```python
from build123d import *

# Parameters (mm, degrees)
SKETCH1_W           = 61
SKETCH1_H           = 101
BOSS_EXTRUDE1_DEPTH = 2
SKETCH2_W           = 65
SKETCH2_H           = 105
BOSS_EXTRUDE2_DEPTH = 2.5
SKETCH4_R           = 3
SKETCH4_R_2         = 1.5
BOSS_EXTRUDE3_DEPTH = 5
SKETCH5_W           = 25
SKETCH5_H           = 32
CUT_EXTRUDE1_DEPTH  = 2
SKETCH6_W           = 2
SKETCH6_H           = 4
CUT_EXTRUDE2_DEPTH  = 3
CUT_EXTRUDE3_DEPTH  = 2.5


with BuildPart() as part:
    # Sketch1 → Boss-Extrude1 (new body)
    with BuildSketch(Plane(origin=(0, 0, 0), x_dir=(1, 0, 0), z_dir=(0, 1, 0))):
        Rectangle(SKETCH1_W, SKETCH1_H)
    extrude(amount=BOSS_EXTRUDE1_DEPTH)

    # Sketch2 → Boss-Extrude2 (add)
    with BuildSketch(Plane(origin=(0, 2, 0), x_dir=(1, 0, 0), z_dir=(0, 1, 0))):
        Rectangle(SKETCH2_W, SKETCH2_H)
    extrude(amount=BOSS_EXTRUDE2_DEPTH)

    # Sketch4 → Boss-Extrude3 (add)
    with BuildSketch(Plane(origin=(0, 4.5, 0), x_dir=(1, 0, 0), z_dir=(0, 1, 0))):
        with Locations((-9, -7.5)):
            Circle(SKETCH4_R)
        with Locations((-9, -7.5)):
            Circle(SKETCH4_R_2, mode=Mode.SUBTRACT)
        with Locations((9, -7.5)):
            Circle(SKETCH4_R)
        with Locations((9, -7.5)):
            Circle(SKETCH4_R_2, mode=Mode.SUBTRACT)
        with Locations((9, 38.5)):
            Circle(SKETCH4_R)
        with Locations((9, 38.5)):
            Circle(SKETCH4_R_2, mode=Mode.SUBTRACT)
        with Locations((-9, 38.5)):
            Circle(SKETCH4_R)
        with Locations((-9, 38.5)):
            Circle(SKETCH4_R_2, mode=Mode.SUBTRACT)
    extrude(amount=BOSS_EXTRUDE3_DEPTH)

    # Sketch5 → Cut-Extrude1 (cut)
    with BuildSketch(Plane(origin=(0, 4.5, 0), x_dir=(1, 0, 0), z_dir=(0, 1, 0))):
        with Locations((0, -48.5)):
            Rectangle(SKETCH5_W, SKETCH5_H)
    extrude(amount=-CUT_EXTRUDE1_DEPTH, mode=Mode.SUBTRACT)

    # Sketch6 → Cut-Extrude2 (cut)
    with BuildSketch(Plane(origin=(0, 9.5, 0), x_dir=(1, 0, 0), z_dir=(0, 1, 0))):
        with Locations((9, -6)):
            Rectangle(SKETCH6_W, SKETCH6_H)
        with Locations((-9, -6)):
            Rectangle(SKETCH6_W, SKETCH6_H)
        with Locations((9, 37)):
            Rectangle(SKETCH6_W, SKETCH6_H)
        with Locations((-9, 37)):
            Rectangle(SKETCH6_W, SKETCH6_H)
    extrude(amount=-CUT_EXTRUDE2_DEPTH, mode=Mode.SUBTRACT)

    # Sketch7 → Cut-Extrude3 (cut)
    with BuildSketch(Plane.XZ):
        Polygon((-16.5, 28.5), (16.5, 28.5), (16.5, 46.5), (26.5, 46.5), (26.5, 28.5), (26.5, -46.5), (-26.5, -46.5), (-26.5, 28.5), (-26.5, 46.5), (-16.5, 46.5), align=None)
    extrude(amount=-CUT_EXTRUDE3_DEPTH, mode=Mode.SUBTRACT)


solid = part.part
```
Work out the finished part from the listing and answer in its coordinate system (mm). A direction names the side the tool comes from. Give positions to 0.01 mm unless a question says otherwise; leave off trailing zeros. Write each loop counter-clockwise with the first axis right and the second up, starting at its lowest first coordinate (ties: lowest second). Pieces come first, ordered by that corner, then holes.
(1) The mould has two halves that part along Z. Classify faces 1 (the flat face through (0, 3, -52.5)), 2 (the flat face through (16.5, 1, 37)), 3 (the flat face through (0, 4, 32.5)), 4 (the flat face through (-10, 9.5, 9)): pulls with the +Z half, pulls with the -Z half, needs draft (parallel to the pull), parting line crosses it, or undercut.
Final values:
face 1: pulls with the -Z half
face 2: undercut
face 3: pulls with the +Z half
face 4: needs draft
(2) Which of the six approach directions +Z, -Z, +X, -X, +Y, -Y give full straight-line access (tool end or side, diameter ignored) to faces 5 (the flat face through (0, 1, -50.5)), 6 (the flat face through (10, 9.5, -40)), 7 (the flat face through (0, 1, 28.5)), 8 (the flat face through (-12.5, 4, 43)), 9 (the cylindrical face through (9, 7, 9))?
Final values:
face 5: -Z, +X, -X, -Y
face 6: +Z, -Z, +X, -X, +Y
face 7: -Y
face 8: +Z, +Y
face 9: +Y
(3) The part is cut by section B-B on x = -21.5. Write down the section's boundary in (y, z), plus the area to 3 significant figures.
Final values:
outline: (0, -50.5) - (2, -50.5) - (2, -52.5) - (4.5, -52.5) - (4.5, 52.5) - (2, 52.5) - (2, 50.5) - (0, 50.5) - (0, 46.5) - (2.5, 46.5) - (2.5, -46.5) - (0, -46.5) - close
area: 232 mm2
(4) Flat-ended cylindrical pins translate along their axes: pin 1 Ø5 at (x, z) = (-9, -38.5) entering from +Y; pin 2 Ø1.2 at (y, z) = (1, 37) entering from +X; pin 3 Ø0.8 at (y, z) = (1.5, 36) entering from -X; pin 4 Ø6 at (x, z) = (21.5, 32) entering from +Y. Find the tip coordinate at first contact, or state that the pin passes through.
Final values:
pin 1: stops at y = 9.5
pin 2: stops at x = 30.5
pin 3: stops at x = -30.5
pin 4: stops at y = 4.5
(5) Straight lines are drawn through the part: line 1 (X direction, y = 6.15, z = -38.5); line 2 (Z direction, x = -9, y = 6.6); line 3 (Z direction, x = -3.5, y = 1.75). For each, find the intervals that lie inside material, in ascending order.
Final values:
line 1: x = -12 to -10.5, -7.5 to -6, 6 to 7.5, 10.5 to 12
line 2: z = -41.5 to -40, 9 to 10.5
line 3: z = -50.5 to -46.5, 28.5 to 50.5
(6) The part is cut by section A-A on y = 1. Write down the section's boundary in (x, z).
Final values:
outline: (-30.5, -50.5) - (30.5, -50.5) - (30.5, 50.5) - (-30.5, 50.5) - close; hole (-26.5, -46.5) - (26.5, -46.5) - (26.5, 46.5) - (16.5, 46.5) - (16.5, 28.5) - (-16.5, 28.5) - (-16.5, 46.5) - (-26.5, 46.5) - close
(7) The part is cut by section C-C on z = -11. Write down the section's boundary in (x, y).
Final values:
outline: (-32.5, 2) - (-30.5, 2) - (-30.5, 0) - (-26.5, 0) - (-26.5, 2.5) - (26.5, 2.5) - (26.5, 0) - (30.5, 0) - (30.5, 2) - (32.5, 2) - (32.5, 4.5) - (-32.5, 4.5) - close
